Job drawing, mm, ordinate dimensions from the low corner. One solid piece. Give positions to 0.01 mm unless a question says otherwise; leave off trailing zeros. Order: outer loops, then holes, each group sorted by start corner. A loop starts at its lowest first (then second) coordinate and runs counter-clockwise, first axis right, second up. Notation, with made-up numbers: (65, -2) -> (113, -2) arc R14 ccw to (113, 22) -> close; hole circle Ø6 at (39.25, 47.25). An arc over 180 degrees is marked (long way). Write item = value, one per line. Start each with the question number.
(1) Saw through at B-B, the plane x = 4. List the corners of the cut face in (y, z), then the cut area to 3 significant figures.
(2) Probe line 1 along X through (y, z) = (7.5, 11); line 2 along Z through (x, y) = (4, 8.25); line 3 along Z through (x, y) = (5, 8.75). List the from-to ranges inside material, lowest first. Write a range as from..to.
(3) Saw through at A-A, the plane z = 43. List the corners of the cut face in (x, y).
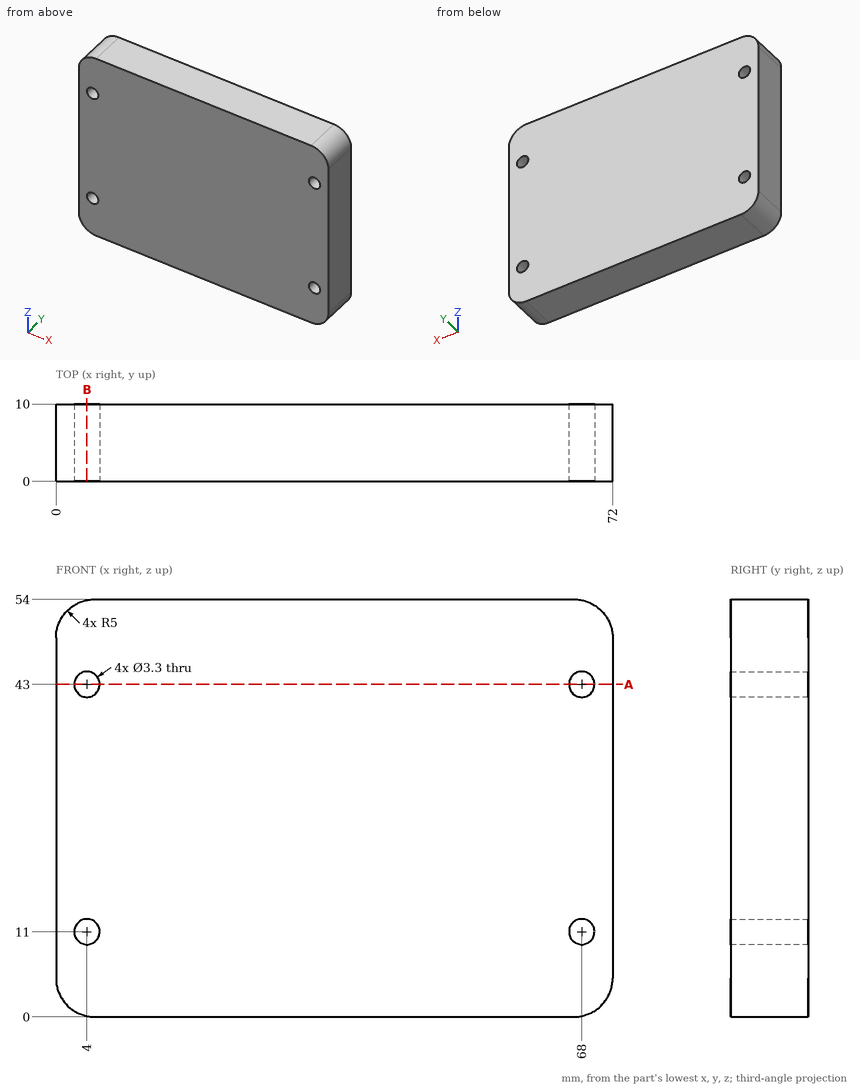
Results list:
q1.outline = (0, 0.1) -> (10, 0.1) -> (10, 9.35) -> (0, 9.35) -> close; (0, 12.65) -> (10, 12.65) -> (10, 41.35) -> (0, 41.35) -> close; (0, 44.65) -> (10, 44.65) -> (10, 53.9) -> (0, 53.9) -> close
q1.area = 472 mm^2
q2.line_1 = 0..2.35, 5.65..66.35, 69.65..72
q2.line_2 = 0.1..9.35, 12.65..41.35, 44.65..53.9
q2.line_3 = 0..9.69, 12.31..41.69, 44.31..54
q3.outline = (0, 0) -> (2.35, 0) -> (2.35, 10) -> (0, 10) -> close; (5.65, 0) -> (66.35, 0) -> (66.35, 10) -> (5.65, 10) -> close; (69.65, 0) -> (72, 0) -> (72, 10) -> (69.65, 10) -> close
